Geometry: final body of the model. Coordinates: model frame, mm. A direction names the side the tool comes from. Give positions to 0.01 mm unless a question says otherwise; leave off trailing zeros. Write each loop counter-clockwise with the first axis right and the second up, starting at its lowest first coordinate (ties: lowest second). Pieces come first, ordered by that corner, then holes. Notation, with made-up numbers: (51.25, 63) -> (92.25, 63) arc R9 ccw to (92.25, 67) -> close; hole circle Ø3 at (33.25, 53). An arc over 180 degrees is marked (long way). Answer in a Markdown table with one row per item. Add a question column.
from build123d import *

# Parameters (mm, degrees)
F1_DEPTH = 63.5
F0_W     = 25.432032
F0_H     = 19.05
F2_DEPTH = 12.7
F3_DEPTH = 7.9375
F5_R     = 6.35


with BuildPart() as f1:
    # F0 (on Front) → F1 (new body, symmetric)
    with BuildSketch(Plane.XZ):
        Polygon((-41.275, -9.525), (41.275, -9.525), (41.275, 9.525), (22.225, 9.525), (-41.275, 9.525), align=None)
    extrude(amount=F1_DEPTH, both=True)

    # F0 (on Front) → F2 (join, symmetric)
    with BuildSketch(Plane.XZ):
        with BuildLine():
            Line((22.225, 9.525), (41.275, 9.525))
            Line((41.275, 9.525), (41.275, 27.0002))
            ThreePointArc((41.275, 27.0002), (45.92468, 38.22552), (57.15, 42.8752))
            Line((57.15, 42.8752), (60.325, 42.8752))
            Line((60.325, 42.8752), (60.325, 61.9252))
            add(Edge.make_bspline(
                [(49.467139, 61.069677), (53.266312, 61.53517), (56.908996, 61.825166), (60.325, 61.9252)],
                knots=[103.848295, 103.848295, 103.848295, 103.848295, 114.316845, 114.316845, 114.316845, 114.316845], degree=3))
            ThreePointArc((49.467139, 61.069677), (29.872907, 48.811111), (22.225, 27.0002))
            Line((22.225, 27.0002), (22.225, 9.525))
        make_face()
        with Locations((73.041016, 52.4002)):
            Rectangle(F0_W, F0_H)
    extrude(amount=F2_DEPTH, both=True)

    # F0 (on Front) → F3 (join, symmetric)
    with BuildSketch(Plane.XZ):
        with BuildLine():
            add(Edge.make_bspline(
                [(-41.275, 9.525), (-41.308278, 34.564084), (11.77924, 56.451974), (49.467139, 61.069677)],
                knots=[0, 0, 0, 0, 103.848295, 103.848295, 103.848295, 103.848295], degree=3))
            Line((-41.275, 9.525), (22.225, 9.525))
            Line((22.225, 9.525), (22.225, 27.0002))
            ThreePointArc((22.225, 27.0002), (29.872907, 48.811111), (49.467139, 61.069677))
        make_face()
    extrude(amount=F3_DEPTH, both=True)

    # F0 (on Front) → F4 (revolve)
    with BuildSketch(Plane.XZ):
        Polygon((85.757032, 66.675), (85.757032, 61.9252), (85.757032, 42.8752), (85.757032, 38.1), (111.125, 38.1), (111.125, 66.675), align=None)
    revolve(axis=Axis((85.757032, 0, 52.3875), (0, 0, -1)))

    # F5
    f5_edges = [f1.edges().sort_by_distance(p)[0] for p in [
        (41.275, -63.5, 0),
        (-41.275, -63.5, 0),
        (-41.275, 63.5, 0),
        (41.275, 63.5, 0),
    ]]
    fillet(f5_edges, radius=F5_R)


solid = f1.part
Q1. Section B-B on y = -33. Return loops of the section in (x, z) (3 decimals), and give its area (3 significant figures).
Q2. Section A-A on z = 3.5. Return loops of the section in (x, y) (3 decimals).
Q3. Contact query for flat-ended pins moving along their axis: pin 1 Ø10 at (x, y) = (-7.5, 0) entering from +Z; pin 2 Ø10 at (x, z) = (74.5, 51) entering from -Y; pin 3 Ø2.5 at (y, z) = (10, 19.5) entering from -X (3 decimals); pin 4 Ø12 at (y, z) = (-32, 31.5) entering from +X. Output: stop coordinate, or through.
Q4. Line query: probe 1 along Y at (x, z) = (4, 44); probe 2 along Z at (x, y) = (8, 23.5) (3 decimals); probe 3 along X at (y, z) = (-2, 25.5) (3 decimals). Output: solid intervals per line, ascending. Write a range as from..to.
Q5. Access query for faces 1 (the flat face through (41.275, -1, 4)), 2 (the flat face through (-5, -7.938, 30)), 3 (the flat face through (22.225, 10, 18)). Directions: +Z, -Z, +X, -X, +Y, -Y. A direction counts if a zero-diameter tool reaches every point of the face in a straight line with its end or side. Return the directions, or none.
Checks:
| question | item | result |
|---|---|---|
| 1 | outline | (-41.275, -9.525) -> (41.275, -9.525) -> (41.275, 9.525) -> (-41.275, 9.525) -> close |
| 1 | area | 1,570 mm^2 |
| 2 | outline | (-41.275, -57.15) arc R6.35 ccw to (-34.925, -63.5) -> (34.925, -63.5) arc R6.35 ccw to (41.275, -57.15) -> (41.275, 57.15) arc R6.35 ccw to (34.925, 63.5) -> (-34.925, 63.5) arc R6.35 ccw to (-41.275, 57.15) -> close |
| 3 | pin 1 | z = 46.54 |
| 3 | pin 2 | y = -24.58 |
| 3 | pin 3 | x = 22.225 |
| 3 | pin 4 | through |
| 4 | probe 1 | -7.94..7.94 |
| 4 | probe 2 | -9.525..9.525 |
| 4 | probe 3 | -34.264..41.275 |
| 5 | face 1 | -Z, +X, +Y, -Y |
| 5 | face 2 | +Z, -X, -Y |
| 5 | face 3 | +Z, -X, +Y |
